Read the model definition and answer for the solid it produces. Units are mm, in the model's axes. A direction names the side the tool comes from. Coordinates: 2 decimals unless noted, no trailing zeros. Loops run counter-clockwise (first coordinate to the right, second up) from the corner with the lowest first, then second, coordinate; pieces in that order, holes last.
Q1. Section B-B (y = 3.05) is taken. Give the vertices of the cut face in (x, z).
Q2. A flat-ended cylindrical pin translates along its axis: P1, Ø2.5, axis at x = 5.5, z = -4.5, coming from the +Y side. Find the tip coordinate at first contact, or state that the pin passes through.
Q3. Section D-D (x = 8) is taken. Give the vertices of the cut face in (y, z), then the cut area to 3 significant figures.
Q4. Section A-A (x = 22.25) is taken. Give the vertices of the cut face in (y, z), then the cut area to 3 significant figures.
Q5. The mould has two halves that part along X. Classify faces 1 (the face through (15, 1, -9)), 2 (the face through (25, 1, -4)), 3 (the face through (5, 1.5, -5)): pulls with the +X half, pulls with the -X half, needs draft (parallel to the pull), parting line crosses it, or undercut.
Q6. Straight lines are drawn through the part: line 1 (Z direction, x = 22.25, y = 0.95); line 2 (X direction, y = 5.05, z = -4.5); line 3 (X direction, y = 0.5, z = -4.5). For each, find the intervals that lie inside material, in ascending order.
Q7. Which of the six approach directions +Z, -Z, +X, -X, +Y, -Y give full straight-line access (tool end or side, diameter ignored) to faces 4 (the face through (5.251, 3.782, -2.115)), 5 (the face through (23.737, 0.739, -4.695))?
Q8. Section C-C (z = -8) is taken. Give the vertices of the cut face in (x, y).
from build123d import *

# Parameters (mm, degrees)
SKETCH2_W               = 25
SKETCH2_H               = 9
BOSS_EXTRUDE3_DEPTH     = 6
SKETCH3_R               = 2.5
CUT_EXTRUDE1_DEPTH      = 4.5
CUT_EXTRUDE2_DEPTH      = 28.239676944
CUT_EXTRUDE2_DEPTH_BACK = 28.239676944
SKETCH4_R               = 1.5
SKETCH5_R               = 1.5
CUT_EXTRUDE3_DEPTH      = 4.5
CUT_EXTRUDE4_DEPTH      = 28.239676944


with BuildPart() as part:
    # Sketch2 → Boss-Extrude3 (new body)
    with BuildSketch(Plane(origin=(0, 0, 0), x_dir=(1, 0, 0), z_dir=(0, 1, 0))):
        with Locations((12.5, 4.5)):
            Rectangle(SKETCH2_W, SKETCH2_H)
    extrude(amount=BOSS_EXTRUDE3_DEPTH)

    # Sketch3 → Cut-Extrude1 (cut)
    with BuildSketch(Plane(origin=(0, 6, 0), x_dir=(1, 0, 0), z_dir=(0, 1, 0))):
        with Locations(Location((4.5, 4.5, 0), (0, 0, 270))):
            Circle(SKETCH3_R)
    extrude(amount=-CUT_EXTRUDE1_DEPTH, mode=Mode.SUBTRACT)

    # Sketch4 → Cut-Extrude2 (cut, two sides: drawn at the far end of the back side and taken through both)
    with BuildSketch(Plane(origin=(0, 6, 0), x_dir=(1, 0, 0), z_dir=(0, 1, 0)).offset(-CUT_EXTRUDE2_DEPTH_BACK)):
        with Locations(Location((22.25, 4.5, 0), (0, 0, 270))):
            Circle(SKETCH4_R)
    extrude(amount=CUT_EXTRUDE2_DEPTH + CUT_EXTRUDE2_DEPTH_BACK, mode=Mode.SUBTRACT)

    # Sketch5 → Cut-Extrude3 (cut)
    with BuildSketch(Plane(origin=(0, 6, 0), x_dir=(1, 0, 0), z_dir=(0, 1, 0))):
        with BuildLine():
            Line((25, 9), (4.5, 9))
            ThreePointArc((4.5, 9), (7.681980515, 7.681980515), (9, 4.5))
            ThreePointArc((9, 4.5), (7.681980515, 1.318019485), (4.5, 0))
            Line((4.5, 0), (25, 0))
            Line((25, 0), (25, 9))
        make_face()
        with Locations(Location((22.25, 4.5, 0), (0, 0, 270))):
            Circle(SKETCH5_R, mode=Mode.SUBTRACT)
    extrude(amount=-CUT_EXTRUDE3_DEPTH, mode=Mode.SUBTRACT)

    # Sketch6 → Cut-Extrude4 (cut, through all)
    with BuildSketch(Plane(origin=(0, 6, 0), x_dir=(1, 0, 0), z_dir=(0, 1, 0))):
        with BuildLine():
            ThreePointArc((0, 4.5), (1.318019485, 7.681980515), (4.5, 9))
            Line((4.5, 9), (0, 9))
            Line((0, 9), (0, 4.5))
        make_face()
        with BuildLine():
            ThreePointArc((4.5, 0), (1.318019485, 1.318019485), (0, 4.5))
            Line((0, 4.5), (0, 0))
            Line((0, 0), (4.5, 0))
        make_face()
    extrude(amount=-CUT_EXTRUDE4_DEPTH, mode=Mode.SUBTRACT)


solid = part.part
Numbers:
1. outline: circle Ø9 at (4.5, -4.5); hole circle Ø5 at (4.5, -4.5)
2. P1: stops at y = 1.5
3. outline: (0, -9) - (1.5, -9) - (1.5, -7.33) - (6, -7.33) - (6, -1.67) - (1.5, -1.67) - (1.5, 0) - (0, 0) - close
3. area: 39.0 mm2
4. outline: (0, -9) - (1.5, -9) - (1.5, -6) - (0, -6) - close; (0, -3) - (1.5, -3) - (1.5, 0) - (0, 0) - close
4. area: 9.00 mm2
5. face 1: needs draft
5. face 2: pulls with the +X half
5. face 3: undercut
6. line 1: z = -9 to -6, -3 to 0
6. line 2: x = 0 to 2, 7 to 9
6. line 3: x = 0 to 20.75, 23.75 to 25
7. face 4: +Y
7. face 5: +Y, -Y
8. outline: (1.67, 0) - (25, 0) - (25, 1.5) - (7.33, 1.5) - (7.33, 6) - (1.67, 6) - close
